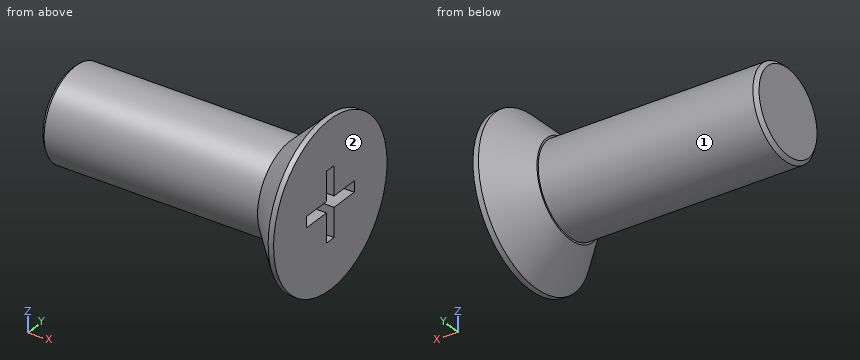
from build123d import *

# Parameters (mm, degrees)
SKETCH_1_R          = 4.5
EXTRUDE_1_DEPTH     = 2.2
SKETCH_2_R          = 2.5
EXTRUDE_3_DEPTH     = 12
CHAMFER_2_SIZE      = 0.2
CHAMFER_3_SIZE      = 1.9
CUT_EXTRUDE_2_DEPTH = 3


with BuildPart() as part:
    # 草图1 → 凸台-拉伸1 (new body)
    with BuildSketch(Plane(origin=(0, 0, 0), x_dir=(0, 0, -1), z_dir=(1, 0, 0))):
        Circle(SKETCH_1_R)
    extrude(amount=EXTRUDE_1_DEPTH)

    # 草图2 → 凸台-拉伸3 (add)
    with BuildSketch(Plane.ZY):
        Circle(SKETCH_2_R)
    extrude(amount=EXTRUDE_3_DEPTH)

    # 倒角2
    chamfer_2_edges = [part.edges().sort_by_distance(p)[0] for p in [
        (-12, 0, -2.5),
    ]]
    chamfer(chamfer_2_edges, length=CHAMFER_2_SIZE)

    # 倒角3
    chamfer_3_edges = [part.edges().sort_by_distance(p)[0] for p in [
        (0, 0, 4.5),
    ]]
    chamfer(chamfer_3_edges, length=CHAMFER_3_SIZE)

    # 草图5 → 切除-拉伸2 (cut)
    with BuildSketch(Plane(origin=(2.2, 0, 0), x_dir=(0, 0, -1), z_dir=(1, 0, 0))):
        Polygon((0.3, 0.3), (1.9, 0.3), (1.9, -0.3), (0.3, -0.3), (0.3, -1.9), (-0.3, -1.9), (-0.3, -0.3), (-1.9, -0.3), (-1.9, 0.3), (-0.3, 0.3), (-0.3, 1.9), (0.3, 1.9), align=None)
    extrude(amount=-CUT_EXTRUDE_2_DEPTH, mode=Mode.SUBTRACT)


solid = part.part
Geometry check sheet. Reference: the model listing, model coordinates, mm. Face numbers are marked on the shaded views. A direction names the side the tool comes from. Round coordinates to 2 decimals unless told otherwise and drop trailing zeros. Loops run counter-clockwise (first coordinate to the right, second up) from the corner with the lowest first, then second, coordinate; pieces in that order, holes last.
Item 1: Gauge pin test, flat ends, axial feed: pin 1 (0.8 mm diameter, centred on x = 0.5, y = -1.5, fed in from -Z); pin 2 (0.5 mm diameter, centred on x = 0.5, y = 0, fed in from +Z); pin 3 (1.3 mm diameter, centred on x = 1, z = -1, fed in from +Y); pin 4 (2 mm diameter, centred on y = 0, z = -1, fed in from +X). Record the tip position at first contact, or that the pin passes through.
Item 2: Thickness scan on line 1 (Y direction, x = -3.5, z = 0); line 2 (Z direction, x = -0.25, y = 1.75); line 3 (X direction, y = 0, z = -1.5). Record the ranges inside material, lowest first.
Item 3: Cross-section at A-A on x = -0.25. Record the boundary of the cut face in (y, z), then the cut area to 3 significant figures.
Item 4: Cross-section at C-C on x = -7. Record the boundary of the cut face in (y, z).
Item 5: Access from +Z, -Z, +X, -X, +Y, -Y to the whole of each face (thin tool, end or side, straight path). Record for the marked faces 1 and 2.
Item 6: Cross-section at B-B on z = 0. Record the boundary of the cut face in (x, y).
Answer sheet:
1. pin 1: stops at z = -3.2
1. pin 2: stops at z = 3.35
1. pin 3: stops at y = 4.15
1. pin 4: stops at x = 2.2
2. line 1: y = -2.5 to 2.5
2. line 2: z = -1.79 to -0.3, 0.3 to 1.79
2. line 3: x = -12 to -0.8
3. outline: circle Ø5 at (0, 0); hole (-1.9, -0.3) - (-0.3, -0.3) - (-0.3, -1.9) - (0.3, -1.9) - (0.3, -0.3) - (1.9, -0.3) - (1.9, 0.3) - (0.3, 0.3) - (0.3, 1.9) - (-0.3, 1.9) - (-0.3, 0.3) - (-1.9, 0.3) - close
3. area: 15.4 mm2
4. outline: circle Ø5 at (0, 0)
5. face 1: -X
5. face 2: +Z, -Z, +X, +Y, -Y
6. outline: (-12, -2.3) - (-11.8, -2.5) - (0, -2.5) - (0, -2.6) - (1.9, -4.5) - (2.2, -4.5) - (2.2, -1.9) - (-0.8, -1.9) - (-0.8, 1.9) - (2.2, 1.9) - (2.2, 4.5) - (1.9, 4.5) - (0, 2.6) - (0, 2.5) - (-11.8, 2.5) - (-12, 2.3) - close
